Autodesk Inventor part; units mm, degrees
ref_plane "YZ Plane" through (0, 0, 0) normal (1, 0, 0) x (0, 1, 0)
ref_plane "XZ Plane" through (0, 0, 0) normal (0, 1, 0) x (-1, 0, 0)
ref_plane "XY Plane" through (0, 0, 0) normal (0, 0, 1) x (1, 0, 0)
sketch "Sketch1" plane through (0, 0, 0) normal (0, 1, 0) x (-1, 0, 0)
  line L0 (25, -22) -> (25, 0)
  line L1 (-25, 0) -> (25, 0)
  line L2 (25, -22) -> (19.05, -22)
  line L3 (19.05, 0) -> (25, 0)
  line L4 (25, 0) -> (25, -22)
  line L5 (-25, -22) -> (-19.05, -22)
  line L6 (-19.05, 0) -> (-25, 0)
  line L7 (-25, 0) -> (-25, -22)
  circle A0 centre (22.025, -11) radius 1.65
  circle A1 centre (-22.025, -11) radius 1.65
  line L8 (25, 0) -> (-25, 0)
  line L9 (-25, 0) -> (-25, -22)
  line L10 (-25, -22) -> (25, -22)
  line L11 (25, -22) -> (25, 0)
  point P0 (0, 0)
  point P1 (22.025, 0)
  point P2 (-25, -11)
  point P3 (0, 0)
  dimension "d2" = 3.3
  dimension "d3" = 3.3
  dimension "d4" = 2.975
  dimension "d5" = 11
  dimension "d6" = 2.975
  dimension "d7" = 11
extrude "Extrusion1" add sketch "Sketch1" along normal blind 2
properties part number "IMU_shin_mount_clamp"
For this review, take the finished solid that the model builds, in its own axes (mm). Give positions to 0.01 mm unless a question says otherwise; leave off trailing zeros. Order: outer loops, then holes, each group sorted by start corner. A loop starts at its lowest first (then second) coordinate and runs counter-clockwise, first axis right, second up. Notation, with made-up numbers: (-30.5, -38.5) - (18.5, -38.5) arc R27 cw to (18.5, -20.5) - close; hole circle Ø8 at (42, -13.75). An arc over 180 degrees is marked (long way). Answer as a JSON object with one key per item and string values. Group by question number.
Item 1: Wall thickness on line 1 along X through (y, z) = (1.1, -10.75); line 2 along X through (y, z) = (1.2, -9.5): over which ranges is each line inside the solid? List them lowest first.
Item 2: Draft analysis for pull direction X (two halves, no side actions). For faces 1 (the flat face through (0, 1, 0)), 2 (the cylindrical face through (-23.55, 0.99, -10.37)), 3 (the flat face through (-25, 1, -11)), state which applies: pulls with the +X half, pulls with the -X half, needs draft (parallel to the pull), parting line crosses it, or undercut.
Item 3: Take a section at B-B on y = 1.6. Give the boundary of the cut face in (x, z) (3 decimals).
Item 4: Take a section at A-A on z = -11. Give the boundary of the cut face in (x, y) (3 decimals), and give its area (3 significant figures).
Reported:
{
 "1": {"line 1": "-25 to -23.66, -20.39 to 20.39, 23.66 to 25", "line 2": "-25 to -22.71, -21.34 to 21.34, 22.71 to 25"},
 "2": {"face 1": "needs draft", "face 2": "undercut", "face 3": "pulls with the -X half"},
 "3": {"outline": "(-25, -22) - (25, -22) - (25, 0) - (-25, 0) - close; hole circle Ø3.3 at (-22.025, -11); hole circle Ø3.3 at (22.025, -11)"},
 "4": {"outline": "(-25, 0) - (-23.675, 0) - (-23.675, 2) - (-25, 2) - close; (-20.375, 0) - (20.375, 0) - (20.375, 2) - (-20.375, 2) - close; (23.675, 0) - (25, 0) - (25, 2) - (23.675, 2) - close", "area": "86.8 mm^2"}
}
